```python
from build123d import *

# Parameters (mm, degrees)
F1_DEPTH = 12.7
F3_D     = 16.66748


with BuildPart() as f1:
    # F0 (on Top) → F1 (new body)
    with BuildSketch(Plane.XY):
        Polygon((22.225, -25.4), (22.225, 25.4), (-22.225, 25.4), (-22.225, -25.4), (-38.1, -25.4), (-38.1, -39.37), (38.1, -39.37), (38.1, -25.4), align=None)
    extrude(amount=F1_DEPTH)

    # F3 (through all)
    with Locations(Plane.XY.offset(12.7)):
        with Locations((0, 0)):
            Hole(F3_D / 2)


solid = f1.part
```
Geometry: final body of the model. Coordinates: model frame, mm. A direction names the side the tool comes from. Coordinates: 2 decimals unless noted, no trailing zeros. Loops run counter-clockwise (first coordinate to the right, second up) from the corner with the lowest first, then second, coordinate; pieces in that order, holes last. Notation, with made-up numbers: M 1.5,13.25 L 14.5,13.25 A32 ccw 14.5,44.25 Z; hole C 38.25,68.5 d8. An arc over 180 degrees is marked long. Put each result on its own line as item: value.
(1) Access query for faces 1 (the face through (30, -25.4, 6)), 2 (the face through (-1, -14, 0)), 3 (the face through (-22.225, 0, 6)). Directions: +Z, -Z, +X, -X, +Y, -Y. A direction counts if a zero-diameter tool reaches every point of the face in a straight line with its end or side. Return the directions, or none.
Answer sheet:
face 1: +Z, -Z, +X, +Y
face 2: -Z, +X, -X, +Y, -Y
face 3: +Z, -Z, -X, +Y
(2) Cut plane B-B on y = 0. Return the cut outline in (x, z) (3 decimals).
Answer sheet:
outline: M -22.225,0 L -8.334,0 L -8.334,12.7 L -22.225,12.7 Z; M 8.334,0 L 22.225,0 L 22.225,12.7 L 8.334,12.7 Z
(3) Material intervals for probe 1 along Y at (x, z) = (0, 7.25); probe 2 along Y at (x, z) = (26.5, 2.25); probe 3 along X at (y, z) = (-18, 8) (3 decimals), sorted ascending.
Answer sheet:
probe 1: y = -39.37 to -8.33, 8.33 to 25.4
probe 2: y = -39.37 to -25.4
probe 3: x = -22.225 to 22.225
(4) Cut plane D-D on y = 18. Return the cut outline in (x, z) (3 decimals).
Answer sheet:
outline: M -22.225,0 L 22.225,0 L 22.225,12.7 L -22.225,12.7 Z
(5) Draft query along Y for faces 4 (the face through (8.326, 0.366, 6.261)), 5 (the face through (0, 25.4, 6)), 6 (the face through (22.225, 0, 6)). Return one class per face: pulls with the +Y half, pulls with the -Y half, needs draft (parallel to the pull), parting line crosses it, or undercut.
Answer sheet:
face 4: undercut
face 5: pulls with the +Y half
face 6: needs draft
(6) First-contact query: pin 1 (2 mm diameter, centred on y = 8.5, z = 6, fed in from -X) (3 decimals); pin 2 (4 mm diameter, centred on y = -4, z = 8, fed in from +X) (3 decimals); pin 3 (6.5 mm diameter, centred on x = 30, z = 6, fed in from +Y). Flat tips, straight axial feed; report the tip coordinate or a pass-through.
Answer sheet:
pin 1: stops at x = -22.225
pin 2: stops at x = 22.225
pin 3: stops at y = -25.4
(7) Cut plane C-C on x = 0. Return the cut outline in (y, z).
Answer sheet:
outline: M -39.37,0 L -8.33,0 L -8.33,12.7 L -39.37,12.7 Z; M 8.33,0 L 25.4,0 L 25.4,12.7 L 8.33,12.7 Z
(8) Cut plane A-A on z = 2.5. Return the cut outline in (x, y) (3 decimals), then the cut area to 3 significant figures.
Answer sheet:
outline: M -38.1,-39.37 L 38.1,-39.37 L 38.1,-25.4 L 22.225,-25.4 L 22.225,25.4 L -22.225,25.4 L -22.225,-25.4 L -38.1,-25.4 Z; hole C 0,0 d16.667
area: 3,100 mm^2
